```python
from build123d import *

# Parameters (mm, degrees)
SKETCH1_R           = 1.6
BOSS_EXTRUDE1_DEPTH = 2


with BuildPart() as part:
    # Sketch1 → Boss-Extrude1 (new body)
    with BuildSketch(Plane(origin=(0, 0, 0), x_dir=(1, 0, 0), z_dir=(0, 1, 0))):
        Polygon((125, 52.071067812), (92.071067812, 85), (-92.071067812, 85), (-125, 52.071067812), (-125, -52.071067812), (-92.071067812, -85), (92.071067812, -85), (125, -52.071067812), align=None)
        with Locations((-89.3372583, -78.4)):
            Circle(SKETCH1_R, mode=Mode.SUBTRACT)
        with Locations((-118.4, -49.3372583)):
            Circle(SKETCH1_R, mode=Mode.SUBTRACT)
        with Locations((-118.4, 49.3372583)):
            Circle(SKETCH1_R, mode=Mode.SUBTRACT)
        with Locations((-89.3372583, 78.4)):
            Circle(SKETCH1_R, mode=Mode.SUBTRACT)
        with Locations((89.3372583, 78.4)):
            Circle(SKETCH1_R, mode=Mode.SUBTRACT)
        with Locations((118.4, 49.3372583)):
            Circle(SKETCH1_R, mode=Mode.SUBTRACT)
        with Locations((118.4, -49.3372583)):
            Circle(SKETCH1_R, mode=Mode.SUBTRACT)
        with Locations((89.3372583, -78.4)):
            Circle(SKETCH1_R, mode=Mode.SUBTRACT)
    extrude(amount=BOSS_EXTRUDE1_DEPTH)


solid = part.part
```
Here's how the part is built. I have some questions about the finished solid (model axes, mm). Give positions to 0.01 mm unless a question says otherwise; leave off trailing zeros. Order: outer loops, then holes, each group sorted by start corner. A loop starts at its lowest first (then second) coordinate and runs counter-clockwise, first axis right, second up. Notation, with made-up numbers: M -2,-27.5 L 40,-27.5 A18 ccw 40,7.5 Z; hole C 30.25,44 d4. An arc over 180 degrees is marked long. Use a Markdown table: item, result. Add a question column.
1. Suppose I cut it at A-A (y = 0.8). Give the number of separate pieces and of enclosed holes in the cut face, and give its area (3 significant figures).
2. I need wall thicknesses on probe 1 along X at (y, z) = (0.55, 78.4); probe 2 along Z at (x, y) = (-118.4, 1.5); probe 3 along Z at (x, y) = (90, 1.2). Which ranges of each line are inside material? Lowest first, please. Write a range as from..to.
3. Suppose I cut it at C-C (x = -109.5). List the corners of the cut face in (y, z) for me.
4. Suppose I cut it at B-B (z = -67). List the corners of the cut face in (x, y) for me, and give its area (3 significant figures).
5. For pin 1 Ø3 at (x, z) = (118.4, 49.34) entering from +Y, with a flat end and sliding along its axis, tell me the tip position at first contact or that it passes through.
Results list:
| question | item | result |
|---|---|---|
| 1 | separate pieces | 1 |
| 1 | enclosed holes | 8 |
| 1 | area | 40,300 mm² |
| 2 | probe 1 | x = -98.67..-90.94, -87.74..87.74, 90.94..98.67 |
| 2 | probe 2 | z = -58.67..-50.94, -47.74..47.74, 50.94..58.67 |
| 2 | probe 3 | z = -85..-79.86, -76.94..76.94, 79.86..85 |
| 3 | outline | M 0,-67.57 L 2,-67.57 L 2,67.57 L 0,67.57 Z |
| 4 | outline | M -110.07,0 L 110.07,0 L 110.07,2 L -110.07,2 Z |
| 4 | area | 440 mm² |
| 5 | pin 1 | passes through |
